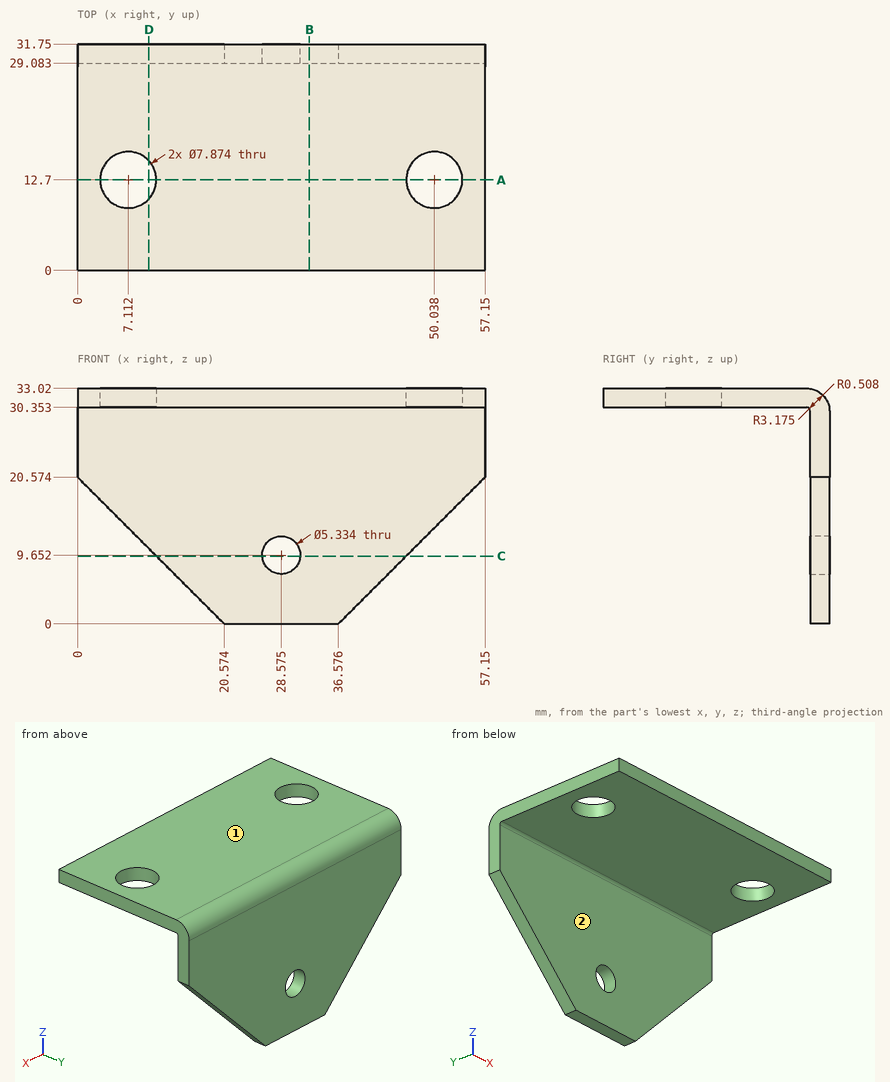
Check sheet for the drawn part. Datum: minimum x, y, z corner. Units: mm. A direction names the side the tool comes from. Coordinates: 2 decimals unless noted, no trailing zeros. Loops run counter-clockwise (first coordinate to the right, second up) from the corner with the lowest first, then second, coordinate; pieces in that order, holes last. Notation, with made-up numbers: (-37.5, -24) -> (-30.5, -24) arc R20 cw to (-30.5, -12) -> close; hole circle Ø9 at (57, 18). An arc over 180 degrees is marked (long way). Answer in a Markdown table with one row per item.
1. Sectioned sample at C-C, the plane z = 9.5. Record the boundary of the cut face in (x, y), then the cut area to 3 significant figures.
Check values:
| item | result |
|---|---|
| outline | (11.07, 29.08) -> (25.91, 29.08) -> (25.91, 31.75) -> (11.07, 31.75) -> close; (31.24, 29.08) -> (46.08, 29.08) -> (46.08, 31.75) -> (31.24, 31.75) -> close |
| area | 79.1 mm2 |
2. Sectioned sample at D-D, the plane x = 10. Record the boundary of the cut face in (y, z) (3 decimals).
Check values:
| item | result |
|---|---|
| outline | (0, 30.353) -> (10.024, 30.353) -> (10.024, 33.02) -> (0, 33.02) -> close; (15.376, 30.353) -> (28.575, 30.353) arc R0.508 cw to (29.083, 29.845) -> (29.083, 10.574) -> (31.75, 10.574) -> (31.75, 29.845) arc R3.175 ccw to (28.575, 33.02) -> (15.376, 33.02) -> close |
3. Material ranges on line 1 along X through (y, z) = (12, 31); line 2 along Z through (x, y) = (46.5, 14.5); line 3 along Y through (x, z) = (8.5, 22), recorded low to high. Write a range as [from, to].
Check values:
| item | result |
|---|---|
| line 1 | x = [0, 3.24], [10.99, 46.16], [53.91, 57.15] |
| line 2 | z = [30.35, 33.02] |
| line 3 | y = [29.08, 31.75] |
4. Go/stop test with a flat-tipped pin: pin 1 (2 mm diameter, centred on x = 39, y = 15, fed in from -Z). Record where the tip stops, or that it passes through.
Check values:
| item | result |
|---|---|
| pin 1 | stops at z = 30.35 |
5. Sectioned sample at B-B, the plane x = 32.5. Record the boundary of the cut face in (y, z) (3 decimals).
Check values:
| item | result |
|---|---|
| outline | (0, 30.353) -> (28.575, 30.353) arc R0.508 cw to (29.083, 29.845) -> (29.083, 0) -> (31.75, 0) -> (31.75, 29.845) arc R3.175 ccw to (28.575, 33.02) -> (0, 33.02) -> close |
6. Access from +Z, -Z, +X, -X, +Y, -Y to the whole of each face (thin tool, end or side, straight path). Record for the marked faces 1 and 2.
Check values:
| item | result |
|---|---|
| face 1 | +Z, +X, -X, +Y, -Y |
| face 2 | -Z, +X, -X, -Y |
7. Sectioned sample at A-A, the plane y = 12.7. Record the boundary of the cut face in (x, z) (3 decimals).
Check values:
| item | result |
|---|---|
| outline | (0, 30.353) -> (3.175, 30.353) -> (3.175, 33.02) -> (0, 33.02) -> close; (11.049, 30.353) -> (46.101, 30.353) -> (46.101, 33.02) -> (11.049, 33.02) -> close; (53.975, 30.353) -> (57.15, 30.353) -> (57.15, 33.02) -> (53.975, 33.02) -> close |
